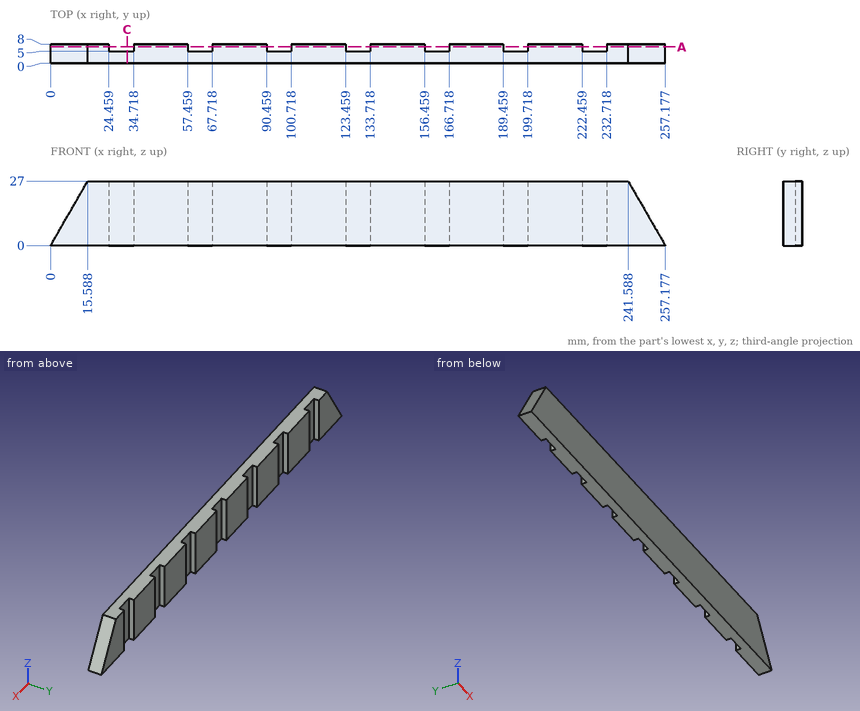
Here's the drawing with two shaded views (mm, measured from the low corner). I have some questions. Coordinates: 2 decimals unless noted, no trailing zeros. Write each loop counter-clockwise with the first axis right and the second up, starting at its lowest first coordinate (ties: lowest second). Pieces come first, ordered by that corner, then holes. Notation, with made-up numbers: M -34.5,5 L -15.5,5 A15 cw -15.5,20 Z; hole C -18.75,-39.75 d1. An arc over 180 degrees is marked long. Write item = value, one per line. Start each with the question number.
Q1. If we section it at A-A, the plane y = 6.75: State how many separate pieces and enclosed holes the cut face has, then the cut area to 3 significant figures.
Q2. If we section it at C-C, the plane x = 32: Write out the boundary of the cut face in (y, z).
Q3. If I drill on L1, parallel to Y at x = 223.5, z = 7.75; L2, parallel to X at y = 2.25, z = 12.25 (1 decimal); L3, parallel to X at y = 3.5, z = 17 (1 decimal), over which ranges is the centre line in solid material (lowest first)? Write a range as [from, to].
Q4. I'm going to push flat-ended pins straight in: pin 1 (1 mm diameter, centred on y = 5.5, z = 24, fed in from +X); pin 2 (1.5 mm diameter, centred on y = 6.5, z = 11, fed in from +X); pin 3 (11.5 mm diameter, centred on x = 229.5, z = 14.5, fed in from +Y); pin 4 (0.9 mm diameter, centred on y = 6.5, z = 19, fed in from +X). Where does each tip first touch, or does it pass through?
Check sheet entries:
q1.separate_pieces = 8
q1.enclosed_holes = 0
q1.area = 4,580 mm²
q2.outline = M 0,0 L 5,0 L 5,27 L 0,27 Z
q3.L1 = [0, 5]
q3.L2 = [7.1, 250.1]
q3.L3 = [9.8, 247.4]
q4.pin_1 = 243.61
q4.pin_2 = 251.26
q4.pin_3 = 8
q4.pin_4 = 246.47
